Can you work these out from the model? Positions are in its coordinate system, mm. Face numbers are marked on the shaded views. Give positions to 0.01 mm unless a question says otherwise; leave off trailing zeros. Loops run counter-clockwise (first coordinate to the right, second up) from the corner with the lowest first, then second, coordinate; pieces in that order, holes last. Notation, with made-up numbers: (89, 62) -> (144, 62) arc R32 cw to (144, 92) -> close; hole circle Ø6 at (-23.5, -14.5). An arc over 180 degrees is marked (long way). Return JSON: item names as keys, results as strings. Group by question number.
Q1. Suppose I cut it at C-C, the plane z = 6.5. Please give me the cut outline in (x, y), and give its area (3 significant figures).
Q2. Suppose I cut it at D-D, the plane y = 19.5. Please give me the cut outline in (x, z), and give its area (3 significant figures).
Q3. Suppose I cut it at B-B, the plane x = 60. Please give me the cut outline in (y, z).
Q4. I need wall thicknesses on line 1 along X through (y, z) = (15.5, 7.75); line 2 along Y through (x, z) = (7, 3); line 3 along Y through (x, z) = (44.5, 3.25). Which ranges of each line are inside material? Lowest first, please. Write a range as [from, to].
Q5. Thinking about a two-plate mould opening in X: for the marked faces 1, 2 and 3, which applies, pulls with the +X half, pulls with the -X half, needs draft (parallel to the pull), parting line crosses it, or undercut?
Q6. Suppose I cut it at A-A, the plane y = 15. Please give me the cut outline in (x, z), and give its area (3 significant figures).
Q7. Will these pins go through, and if not, where does the flat tip stop? pin 1 (4 mm diameter, centred on x = 59.5, z = 6, fed in from -Y); pin 2 (1 mm diameter, centred on y = 10, z = 5.5, fed in from -X).
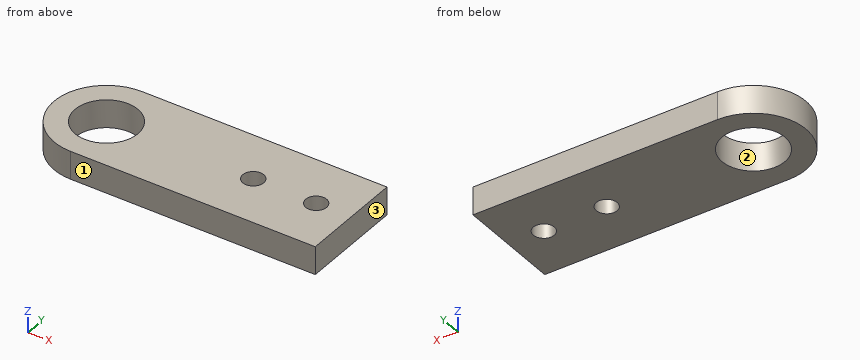
```python
from build123d import *

# Parameters (mm, degrees)
BOSS_EXTRUDE1_DEPTH   = 8
CUT_EXTRUDE1_REACH    = 78.577
SKETCH2_R             = 9
F_6_0MM_DOWEL_HOLE1_D = 6


with BuildPart() as part:
    # Sketch1 → Boss-Extrude1 (new body)
    with BuildSketch(Plane.XY):
        with BuildLine():
            Line((0, 0), (70, 0))
            Line((70, 0), (70, 30))
            Line((70, 30), (0, 30))
            ThreePointArc((0, 30), (-15, 15), (0, 0))
        make_face()
    extrude(amount=BOSS_EXTRUDE1_DEPTH)

    # Sketch2 → Cut-Extrude1 (cut, up to next)
    with BuildSketch(Plane.XY.offset(8), mode=Mode.PRIVATE) as cut_extrude1_sk1:
        with Locations((0, 15)):
            Circle(SKETCH2_R)
    cut_extrude1_tool1 = extrude(cut_extrude1_sk1.sketch, amount=-CUT_EXTRUDE1_REACH, mode=Mode.PRIVATE) & part.part
    add(cut_extrude1_tool1.solids().sort_by_distance((0, 15, 8))[0], mode=Mode.SUBTRACT)

    # Ø6.0mm Dowel Hole1 (through all)
    with Locations(Plane(origin=(0, 0, 0), x_dir=(-1, 0, 0), z_dir=(0, 0, -1))):
        with Locations((-42, 15), (-60, 15)):
            Hole(F_6_0MM_DOWEL_HOLE1_D / 2)


solid = part.part
```
Ans:
{
 "1": {"outline": "(0, 0) -> (70, 0) -> (70, 30) -> (0, 30) arc R15 ccw to start; hole circle Ø18 at (0, 15); hole circle Ø6 at (42, 15); hole circle Ø6 at (60, 15)", "area": "2,140 mm^2"},
 "2": {"outline": "(-14.31, 0) -> (-7.79, 0) -> (-7.79, 8) -> (-14.31, 8) -> close; (7.79, 0) -> (70, 0) -> (70, 8) -> (7.79, 8) -> close", "area": "550 mm^2"},
 "3": {"outline": "(0, 0) -> (12, 0) -> (12, 8) -> (0, 8) -> close; (18, 0) -> (30, 0) -> (30, 8) -> (18, 8) -> close"},
 "4": {"line 1": "x = [-14.99, -8.99], [8.99, 39.04], [44.96, 57.04], [62.96, 70]", "line 2": "y = [0, 9.34], [20.66, 30]", "line 3": "y = [0, 13.34], [16.66, 30]"},
 "5": {"face 1": "needs draft", "face 2": "undercut", "face 3": "pulls with the +X half"},
 "6": {"outline": "(-15, 0) -> (-9, 0) -> (-9, 8) -> (-15, 8) -> close; (9, 0) -> (39, 0) -> (39, 8) -> (9, 8) -> close; (45, 0) -> (57, 0) -> (57, 8) -> (45, 8) -> close; (63, 0) -> (70, 0) -> (70, 8) -> (63, 8) -> close", "area": "440 mm^2"},
 "7": {"pin 1": "stops at y = 0", "pin 2": "stops at x = -14.31"}
}
